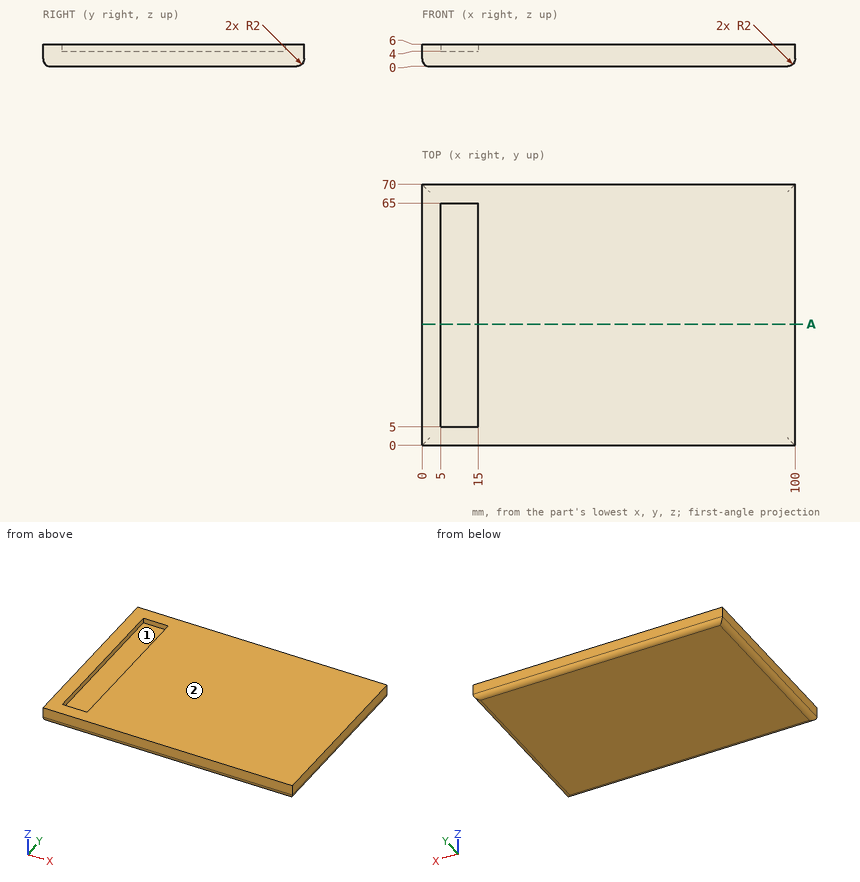
For this review, use the dimensioned drawing (mm, ordinates from the lowest corner) and the shaded views. Round coordinates to 2 decimals unless told otherwise and drop trailing zeros. Write each loop counter-clockwise with the first axis right and the second up, starting at its lowest first coordinate (ties: lowest second). Pieces come first, ordered by that corner, then holes. Notation, with made-up numbers: M 31.5,-2.5 L 57.5,-2.5 A11 cw 57.5,14.5 Z; hole C 8,-12.5 d6. An arc over 180 degrees is marked long. Write item = value, one per line. Start each with the question number.
(1) For line 1 along X through (y, z) = (15, 5.6); line 2 along Y through (x, z) = (10, 0.2); line 3 along X through (y, z) = (26, 1.6), list the stretches that pass through material, from the lowest coordinate up.
(2) Clearance check with flat-ended pins moving along their axes: pin 1 Ø3 at (x, z) = (63, 3.5) entering from -Y; pin 2 Ø3 at (x, y) = (9.5, 28) entering from +Z. State where each tip first meets the part, or that it passes through.
(3) We need section A-A (y = 32.5). Give the boundary of the cut face in (x, z), then the cut area to 3 significant figures.
(4) The part is to be moulded in two halves that separate along Y. For the marked faces 1 and 2, say which applies: +Y half, -Y half, draft (parallel to the pull), parting line (faces both ways), or undercut.
Results found:
q1.line_1 = 0 to 5, 15 to 100
q1.line_2 = 1.13 to 68.87
q1.line_3 = 0.04 to 99.96
q2.pin_1 = 0
q2.pin_2 = 4
q3.outline = M 0,2 A2 ccw 2,0 L 98,0 A2 ccw 100,2 L 100,6 L 15,6 L 15,4 L 5,4 L 5,6 L 0,6 Z
q3.area = 578 mm²
q4.face_1 = undercut
q4.face_2 = draft
